```python
from build123d import *

# Parameters (mm, degrees)
BOSS_EXTRUDE1_DEPTH = 2.54
CUT_EXTRUDE2_DEPTH  = 3.683
CUT_EXTRUDE4_START  = 10.16
CUT_EXTRUDE4_DEPTH  = 3.683
SKETCH2_W           = 2.286
SKETCH2_H           = 14.478
BOSS_EXTRUDE2_DEPTH = 2.794
SKETCH3_W           = 1.143
SKETCH3_H           = 1.016
CUT_EXTRUDE5_DEPTH  = 0.254
DRAFT2_START        = 5.334
DRAFT2_DEPTH        = 14.478
DRAFT2_2_DEPTH      = 9.398
CUT_EXTRUDE6_DEPTH  = 23.895250599


# Read off the part's stored shape, not the designer's step: Draft2
with BuildPart() as part:
    # Model → Boss-Extrude1 (new body)
    with BuildSketch(Plane.XY):
        with BuildLine():
            Line((2.794, 15.748), (7.366, 15.748))
            Line((7.366, 15.748), (7.366, 14.732))
            Line((7.366, 14.732), (6.223, 14.732))
            Line((6.223, 14.732), (6.223, 5.334))
            Line((6.223, 5.334), (10.16, 5.334))
            Line((10.16, 5.334), (10.16, 1.650767887))
            ThreePointArc((10.16, 1.650767887), (9.722993685, 0.582582169), (8.662597467, 0.127))
            Line((8.662597467, 0.127), (3.572534178, 0.038152615))
            ThreePointArc((3.572534178, 0.038152615), (3.219068772, -0.113708108), (3.0734, -0.469770014))
            Line((3.0734, -0.469770014), (3.0734, -0.741620434))
            ThreePointArc((3.0734, -0.741620434), (2.5654, -1.249620434), (2.0574, -0.741620434))
            Line((2.0574, -0.741620434), (2.0574, -0.469770014))
            ThreePointArc((2.0574, -0.469770014), (2.494406315, 0.598415704), (3.554802533, 1.053997873))
            Line((3.554802533, 1.053997873), (8.644865822, 1.142845258))
            ThreePointArc((8.644865822, 1.142845258), (8.998331228, 1.294705981), (9.144, 1.650767887))
            Line((9.144, 1.650767887), (9.144, 3.556))
            Line((9.144, 3.556), (1.016, 3.556))
            Line((1.016, 3.556), (1.016, 0))
            Line((1.016, 0), (0, 0))
            Line((0, 0), (0, 5.334))
            Line((0, 5.334), (3.937, 5.334))
            Line((3.937, 5.334), (3.937, 14.732))
            Line((3.937, 14.732), (2.794, 14.732))
            Line((2.794, 14.732), (2.794, 15.748))
        make_face()
    extrude(amount=-BOSS_EXTRUDE1_DEPTH)

    # Sketch1 → Cut-Extrude2 (cut)
    with BuildSketch(Plane(origin=(0, 0, 0), x_dir=(0, 0, -1), z_dir=(1, 0, 0))):
        Polygon((0, 5.334), (2.54, 5.334), (2.54, 3.555472853), align=None)
    extrude(amount=CUT_EXTRUDE2_DEPTH, mode=Mode.SUBTRACT)

    # Sketch1<3> → Cut-Extrude4 (cut)
    with BuildSketch(Plane(origin=(0, 0, 0), x_dir=(0, 0, -1), z_dir=(1, 0, 0)).offset(CUT_EXTRUDE4_START)):
        Polygon((0, 5.334), (2.54, 5.334), (2.54, 3.555472853), align=None)
    extrude(amount=-CUT_EXTRUDE4_DEPTH, mode=Mode.SUBTRACT)

    # Sketch2 → Boss-Extrude2 (add)
    with BuildSketch(Plane(origin=(0, 0, -2.54), x_dir=(-1, 0, 0), z_dir=(0, 0, -1))):
        with Locations((-5.08, 12.573)):
            Rectangle(SKETCH2_W, SKETCH2_H)
    extrude(amount=BOSS_EXTRUDE2_DEPTH)

    # Sketch3 → Cut-Extrude5 (cut)
    with BuildSketch(Plane(origin=(0, 0, -2.54), x_dir=(-1, 0, 0), z_dir=(0, 0, -1))):
        with Locations((-6.7945, 15.24)):
            Rectangle(SKETCH3_W, SKETCH3_H)
        with Locations((-3.3655, 15.24)):
            Rectangle(SKETCH3_W, SKETCH3_H)
    extrude(amount=-CUT_EXTRUDE5_DEPTH, mode=Mode.SUBTRACT)

    # Draft2 outline → Draft2 (cut)
    with BuildSketch(Plane(origin=(0, 0, 0), x_dir=(1, 0, 0), z_dir=(0, 1, 0)).offset(DRAFT2_START)):
        Polygon((4.216543095, 5.334), (3.937, 5.334), (3.937, 2.286), (4.056804183, 2.286), align=None)
        Polygon((6.223, 5.334), (5.943456905, 5.334), (6.103195817, 2.286), (6.223, 2.286), align=None)
    extrude(amount=DRAFT2_DEPTH, mode=Mode.SUBTRACT)

    # Draft2 2 outline → Draft2 2 (cut)
    with BuildSketch(Plane(origin=(0, 0, 0), x_dir=(1, 0, 0), z_dir=(0, 1, 0)).offset(DRAFT2_START)):
        Polygon((3.937, 0), (4.056804184, 2.286), (3.937, 2.286), align=None)
        Polygon((6.223, 2.286), (6.103195817, 2.286), (6.223, 0), align=None)
    extrude(amount=DRAFT2_2_DEPTH, mode=Mode.SUBTRACT)

    # Sketch4 → Cut-Extrude6 (cut, through all)
    with BuildSketch(Plane(origin=(0, 0, 0), x_dir=(0, 0, -1), z_dir=(1, 0, 0))):
        with BuildLine():
            ThreePointArc((4.953, 19.812), (5.222407684, 19.700407684), (5.334, 19.431))
            Line((5.334, 19.431), (5.334, 19.812))
            Line((5.334, 19.812), (4.953, 19.812))
        make_face()
        with BuildLine():
            ThreePointArc((4.953, 18.288), (5.222407684, 18.176407684), (5.334, 17.907))
            Line((5.334, 17.907), (5.334, 19.431))
            ThreePointArc((5.334, 19.431), (5.222407684, 19.161592316), (4.953, 19.05))
            ThreePointArc((4.953, 19.05), (4.683592316, 18.938407684), (4.572, 18.669))
            ThreePointArc((4.572, 18.669), (4.683592316, 18.399592316), (4.953, 18.288))
        make_face()
        with BuildLine():
            ThreePointArc((4.953, 16.764), (5.222407684, 16.652407684), (5.334, 16.383))
            Line((5.334, 16.383), (5.334, 17.907))
            ThreePointArc((5.334, 17.907), (5.222407684, 17.637592316), (4.953, 17.526))
            ThreePointArc((4.953, 17.526), (4.683592316, 17.414407684), (4.572, 17.145))
            ThreePointArc((4.572, 17.145), (4.683592316, 16.875592316), (4.953, 16.764))
        make_face()
        with BuildLine():
            ThreePointArc((4.953, 15.24), (5.222407684, 15.128407684), (5.334, 14.859))
            Line((5.334, 14.859), (5.334, 16.383))
            ThreePointArc((5.334, 16.383), (5.222407684, 16.113592316), (4.953, 16.002))
            ThreePointArc((4.953, 16.002), (4.683592316, 15.890407684), (4.572, 15.621))
            ThreePointArc((4.572, 15.621), (4.683592316, 15.351592316), (4.953, 15.24))
        make_face()
        with BuildLine():
            ThreePointArc((4.953, 13.716), (5.222407684, 13.604407684), (5.334, 13.335))
            Line((5.334, 13.335), (5.334, 14.859))
            ThreePointArc((5.334, 14.859), (5.222407684, 14.589592316), (4.953, 14.478))
            ThreePointArc((4.953, 14.478), (4.683592316, 14.366407684), (4.572, 14.097))
            ThreePointArc((4.572, 14.097), (4.683592316, 13.827592316), (4.953, 13.716))
        make_face()
        with BuildLine():
            ThreePointArc((4.953, 12.192), (5.222407684, 12.080407684), (5.334, 11.811))
            Line((5.334, 11.811), (5.334, 13.335))
            ThreePointArc((5.334, 13.335), (5.222407684, 13.065592316), (4.953, 12.954))
            ThreePointArc((4.953, 12.954), (4.683592316, 12.842407684), (4.572, 12.573))
            ThreePointArc((4.572, 12.573), (4.683592316, 12.303592316), (4.953, 12.192))
        make_face()
        with BuildLine():
            ThreePointArc((4.953, 10.668), (5.222407684, 10.556407684), (5.334, 10.287))
            Line((5.334, 10.287), (5.334, 11.811))
            ThreePointArc((5.334, 11.811), (5.222407684, 11.541592316), (4.953, 11.43))
            ThreePointArc((4.953, 11.43), (4.683592316, 11.318407684), (4.572, 11.049))
            ThreePointArc((4.572, 11.049), (4.683592316, 10.779592316), (4.953, 10.668))
        make_face()
        with BuildLine():
            ThreePointArc((4.953, 9.144), (5.222407684, 9.032407684), (5.334, 8.763))
            Line((5.334, 8.763), (5.334, 10.287))
            ThreePointArc((5.334, 10.287), (5.222407684, 10.017592316), (4.953, 9.906))
            ThreePointArc((4.953, 9.906), (4.683592316, 9.794407684), (4.572, 9.525))
            ThreePointArc((4.572, 9.525), (4.683592316, 9.255592316), (4.953, 9.144))
        make_face()
        with BuildLine():
            ThreePointArc((4.953, 7.62), (5.222407684, 7.508407684), (5.334, 7.239))
            Line((5.334, 7.239), (5.334, 8.763))
            ThreePointArc((5.334, 8.763), (5.222407684, 8.493592316), (4.953, 8.382))
            ThreePointArc((4.953, 8.382), (4.683592316, 8.270407684), (4.572, 8.001))
            ThreePointArc((4.572, 8.001), (4.683592316, 7.731592316), (4.953, 7.62))
        make_face()
        with BuildLine():
            ThreePointArc((4.572, 6.477), (4.683592316, 6.207592316), (4.953, 6.096))
            Line((4.953, 6.096), (4.953, 3.556))
            Line((4.953, 3.556), (5.334, 3.556))
            Line((5.334, 3.556), (5.334, 7.239))
            ThreePointArc((5.334, 7.239), (5.222407684, 6.969592316), (4.953, 6.858))
            ThreePointArc((4.953, 6.858), (4.683592316, 6.746407684), (4.572, 6.477))
        make_face()
    extrude(amount=CUT_EXTRUDE6_DEPTH, mode=Mode.SUBTRACT)


solid = part.part
```
For this review, take the finished solid that the model builds, in its own axes (mm). A direction names the side the tool comes from. Coordinates: 2 decimals unless noted, no trailing zeros. Write each loop counter-clockwise with the first axis right and the second up, starting at its lowest first coordinate (ties: lowest second). Pieces come first, ordered by that corner, then holes. Notation, with made-up numbers: (-24.5, 85) - (-7.5, 85) arc R8 ccw to (-7.5, 95) - close; hole circle Ø4 at (57.25, -2.75). An arc over 180 degrees is marked (long way). Put each result on its own line as item: value.
1. Wall thickness on probe 1 along Y at (x, z) = (3.75, -1.7); probe 2 along Y at (x, z) = (5.75, -4.4); probe 3 along X at (y, z) = (12.25, -4.6): over which ranges is each line inside the solid? List them lowest first.
Values found:
probe 1: 0.04 to 1.06, 3.56 to 5.33, 14.73 to 15.75
probe 2: 5.33 to 19.81
probe 3: 4.18 to 5.98
2. For pin 1 (2 mm diameter, centred on y = 1, z = -1, fed in from +X); pin 2 (1 mm diameter, centred on y = 7.5, z = -1, fed in from +X); pin 3 (2 mm diameter, centred on y = 14, z = -4, fed in from +X); pin 4 (1.6 mm diameter, centred on x = 5, z = -4, fed in from -Y), all flat-tipped, find the tip position at first contact; note any pin that passes through.
Values found:
pin 1: x = 10.16
pin 2: x = 6.2
pin 3: x = 6.07
pin 4: y = 5.33
3. Add section A-A, the plane x = 6.75. Give the boundary of the cut face in (y, z), then the cut area to 3 significant figures.
Values found:
outline: (0.09, -2.54) - (1.11, -2.54) - (1.11, 0) - (0.09, 0) - close; (3.56, -2.54) - (5.33, 0) - (3.56, 0) - close; (14.73, -2.29) - (15.75, -2.29) - (15.75, 0) - (14.73, 0) - close
area: 7.16 mm²
4. Add section D-D, the plane x = 2.25. Give the boundary of the cut face in (y, z), then the cut area to 3 significant figures.
Values found:
outline: (-1.14, -2.54) - (0.27, -2.54) - (0.27, 0) - (-1.14, 0) - close; (3.56, -2.54) - (5.33, 0) - (3.56, 0) - close
area: 5.84 mm²
5. Machinability: for faces 4 (the flat face through (5, 15.748, -1)), 5 (the flat face through (0.5, 0, -1.3)), 6 (the flat face through (3, 15, -2.286)), which of the approach directions +Z, -Z, +X, -X, +Y, -Y give a long, thin tool a straight path to every point of the face, cutting with its end or side? Answer none if there is none.
Values found:
face 4: +Z, +X, -X, +Y
face 5: +Z, -Z, -X, -Y
face 6: -Z, -X, +Y
6. Mouldability with a two-part tool opening along X and no side actions: class faces 1 (the cylindrical face through (9.73, 0.59, -1.25)), 2 (the flat face through (1.016, 2, -1)), 3 (the flat face through (0.5, 1.8, -2.54)) as released by +X, released by -X, zero draft, split by the parting line, or undercut.
Values found:
face 1: released by +X
face 2: undercut
face 3: zero draft
7. Add section C-C, the plane z = -0.75. Give the boundary of the cut face in (x, y), then the cut area to 3 significant figures.
Values found:
outline: (0, 0) - (1.02, 0) - (1.02, 3.56) - (9.14, 3.56) - (9.14, 1.65) arc R0.51 cw to (8.64, 1.14) - (3.55, 1.05) arc R1.52 ccw to (2.06, -0.47) - (2.06, -0.74) arc R0.51 ccw to (3.07, -0.74) - (3.07, -0.47) arc R0.51 cw to (3.57, 0.04) - (8.66, 0.13) arc R1.52 ccw to (10.16, 1.65) - (10.16, 4.81) - (6.48, 4.81) - (6.48, 5.33) - (6.18, 5.33) - (6.18, 14.73) - (7.37, 14.73) - (7.37, 15.75) - (2.79, 15.75) - (2.79, 14.73) - (3.98, 14.73) - (3.98, 5.33) - (3.68, 5.33) - (3.68, 4.81) - (0, 4.81) - close
area: 54.2 mm²
8. Add section B-B, the plane y = 4. Give the boundary of the cut face in (x, z).
Values found:
outline: (0, -1.91) - (3.68, -1.91) - (3.68, -2.54) - (6.48, -2.54) - (6.48, -1.91) - (10.16, -1.91) - (10.16, 0) - (0, 0) - close
